from build123d import *

# Parameters (mm, degrees)
SKETCH1_W           = 42
SKETCH1_H           = 22
BOSS_EXTRUDE1_DEPTH = 16
SHELL2_T            = -4


with BuildPart() as part:
    # Sketch1 → Boss-Extrude1 (new body)
    with BuildSketch(Plane(origin=(0, 0, 0), x_dir=(1, 0, 0), z_dir=(0, 1, 0))):
        with Locations((2.633773294, 1.402399006)):
            Rectangle(SKETCH1_W, SKETCH1_H)
    extrude(amount=BOSS_EXTRUDE1_DEPTH)

    # Shell2
    shell2_openings = [part.faces().sort_by_distance(p)[0] for p in [
        (2.633773294, 0, -1.402399006),
        (2.633773294, 8, -12.402399006),
        (2.633773294, 8, 9.597600994),
    ]]
    offset(amount=SHELL2_T, openings=shell2_openings, kind=Kind.INTERSECTION)


solid = part.part
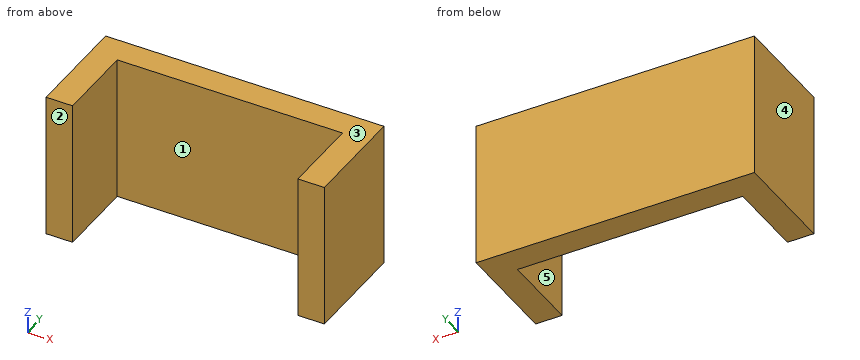
Input: part model. Units: mm. Frame: model coordinates. Face numbers are marked on the shaded views. A direction names the side the tool comes from. Coordinates: 2 decimals unless noted, no trailing zeros. Order: outer loops, then holes, each group sorted by start corner. A loop starts at its lowest first (then second) coordinate and runs counter-clockwise, first axis right, second up.
1. Cut plane C-C, the plane x = 10. Return loops of the section in (y, z), plus the area to 3 significant figures.
Checked values:
outline: (12, -12.4) - (16, -12.4) - (16, 9.6) - (12, 9.6) - close
area: 88.0 mm2
2. Cut plane A-A, the plane y = 7.75. Return loops of the section in (x, z), plus the area to 3 significant figures.
Checked values:
outline: (-18.37, -12.4) - (-14.37, -12.4) - (-14.37, 9.6) - (-18.37, 9.6) - close; (19.63, -12.4) - (23.63, -12.4) - (23.63, 9.6) - (19.63, 9.6) - close
area: 176 mm2
3. Draft query along X for the marked faces 3, 4 and 5. Return one class per face: +X half, -X half, draft (parallel to the pull), parting line (faces both ways), or undercut.
Checked values:
face 3: draft
face 4: -X half
face 5: undercut
4. Access query for the marked faces 1 and 2. Directions: +Z, -Z, +X, -X, +Y, -Y. A direction counts if a zero-diameter tool reaches every point of the face in a straight line with its end or side. Return the directions, or none.
Checked values:
face 1: +Z, -Z, -Y
face 2: +Z, -Z, +X, -X, -Y
5. Ray query, line 1 along X through (y, z) = (4.5, -5.75); line 2 along Y through (x, z) = (5.5, -11). Return the intervals inside material, ascending.
Checked values:
line 1: x = -18.37 to -14.37, 19.63 to 23.63
line 2: y = 12 to 16
6. Contact query for a flat-ended pin moving along its axis: P1, Ø8, axis at x = -4.5, z = -8.5, coming from the -Y side. Output: stop coordinate, or through.
Checked values:
P1: stops at y = 12
7. Cut plane B-B, the plane z = 5.25. Return loops of the section in (x, y).
Checked values:
outline: (-18.37, 0) - (-14.37, 0) - (-14.37, 12) - (19.63, 12) - (19.63, 0) - (23.63, 0) - (23.63, 16) - (-18.37, 16) - close
